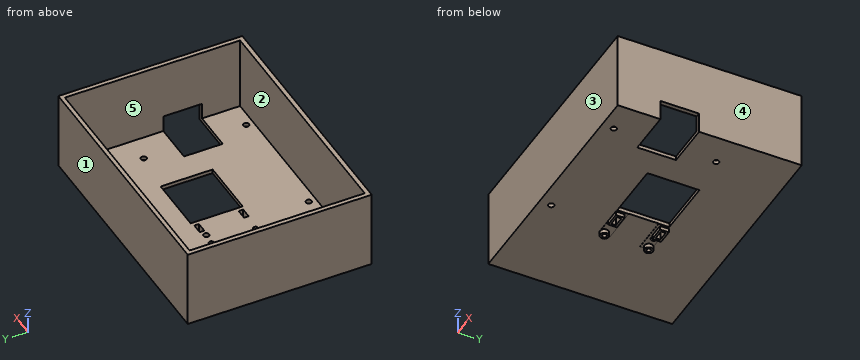
from build123d import *

# Parameters (mm, degrees)
SKETCH_1_W          = 120
SKETCH_1_H          = 80
EXTRUDE_1_DEPTH     = 38
SKETCH_3_W          = 117.6
SKETCH_3_H          = 77.6
CUT_EXTRUDE_1_DEPTH = 36
SKETCH_4_W          = 25.152970524
SKETCH_4_H          = 18.492901276
CUT_EXTRUDE_2_DEPTH = 10
SKETCH_7_W          = 17.413678367
SKETCH_7_H          = 5.076618726
SKETCH_7_H_2        = 5.541721388
EXTRUDE_2_DEPTH     = 0.1
SKETCH_9_W          = 27.882777132
SKETCH_9_H          = 24.878568111
CUT_EXTRUDE_4_DEPTH = 12
SKETCH_12_R         = 1.085209003
SKETCH_12_R_2       = 1.1
SKETCH_12_W         = 5.025
SKETCH_12_H         = 2.2
CUT_EXTRUDE_5_DEPTH = 12
SKETCH_13_R         = 1.35
CUT_EXTRUDE_6_DEPTH = 12
SKETCH_14_W         = 117.6
SKETCH_14_H         = 36
CUT_EXTRUDE_7_DEPTH = 10
EXTRUDE_3_DEPTH     = 5
SKETCH_16_W         = 120
SKETCH_16_H         = 38
EXTRUDE_4_DEPTH     = 2
SKETCH_17_W         = 36
SKETCH_17_H         = 83.8
EXTRUDE_5_DEPTH     = 1
EXTRUDE_6_DEPTH     = 1
SKETCH_19_W         = 120
SKETCH_19_H         = 38
EXTRUDE_7_DEPTH     = 1
EXTRUDE_START       = 2
SKETCH_20_R         = 2
SKETCH_20_R_2       = 1.085209003
SKETCH_20_R_3       = 2.001649737
SKETCH_20_R_4       = 1.1
SKETCH_20_W         = 7.2
SKETCH_20_H         = 4.2
SKETCH_20_W_2       = 5.025
SKETCH_20_H_2       = 2.2
EXTRUDE_8_DEPTH     = 2


with BuildPart() as part:
    # 草图1 → 凸台-拉伸1 (new body)
    with BuildSketch(Plane.XY):
        with Locations((-463.106796117, 303.186737633)):
            Rectangle(SKETCH_1_W, SKETCH_1_H)
    extrude(amount=EXTRUDE_1_DEPTH)

    # 草图3 → 切除-拉伸1 (cut)
    with BuildSketch(Plane.XY.offset(38)):
        with Locations((-463.106796117, 303.186737633)):
            Rectangle(SKETCH_3_W, SKETCH_3_H)
    extrude(amount=-CUT_EXTRUDE_1_DEPTH, mode=Mode.SUBTRACT)

    # 草图4 → 切除-拉伸2 (cut)
    with BuildSketch(Plane(origin=(0, 0, 0), x_dir=(-1, 0, 0), z_dir=(0, 0, -1))):
        with Locations((411.924701676, 291.841861287)):
            Rectangle(SKETCH_4_W, SKETCH_4_H)
    extrude(amount=-CUT_EXTRUDE_2_DEPTH, mode=Mode.SUBTRACT)

    # 草图7 → 凸台-拉伸2 (add)
    with BuildSketch(Plane(origin=(0, 0, 0), x_dir=(-1, 0, 0), z_dir=(0, 0, -1))):
        with Locations((474.461956934, 316.64842827)):
            Rectangle(SKETCH_7_W, SKETCH_7_H)
        with Locations((474.461956934, 296.957598327)):
            Rectangle(SKETCH_7_W, SKETCH_7_H_2)
    extrude(amount=EXTRUDE_2_DEPTH)

    # 草图9 → 切除-拉伸4 (cut)
    with BuildSketch(Plane(origin=(0, 0, 0), x_dir=(-1, 0, 0), z_dir=(0, 0, -1))):
        with Locations((451.813729184, 306.747453577)):
            Rectangle(SKETCH_9_W, SKETCH_9_H)
    extrude(amount=-CUT_EXTRUDE_4_DEPTH, mode=Mode.SUBTRACT)

    # 草图12 → 切除-拉伸5 (cut)
    with BuildSketch(Plane(origin=(0, 0, -0.1), x_dir=(-1, 0, 0), z_dir=(0, 0, -1))):
        with Locations((481.368796117, 317.386737633)):
            Circle(SKETCH_12_R)
        with Locations((481.368796117, 296.186737633)):
            Circle(SKETCH_12_R_2)
        with Locations((470.281296117, 317.386737633)):
            Rectangle(SKETCH_12_W, SKETCH_12_H)
        with Locations((470.281296117, 296.186737633)):
            Rectangle(SKETCH_12_W, SKETCH_12_H)
    extrude(amount=-CUT_EXTRUDE_5_DEPTH, mode=Mode.SUBTRACT)

    # 草图13 → 切除-拉伸6 (cut)
    with BuildSketch(Plane.XY.offset(2)):
        with Locations((-475.806796117, 316.886737633)):
            Circle(SKETCH_13_R)
        with Locations((-417.806796117, 316.886737633)):
            Circle(SKETCH_13_R)
        with Locations((-417.806796117, 267.886737633)):
            Circle(SKETCH_13_R)
        with Locations((-475.806796117, 267.886737633)):
            Circle(SKETCH_13_R)
    extrude(amount=-CUT_EXTRUDE_6_DEPTH, mode=Mode.SUBTRACT)

    # 草图14 → 切除-拉伸7 (cut)
    with BuildSketch(Plane.XZ.offset(-341.986737633)):
        with Locations((-463.106796117, 20)):
            Rectangle(SKETCH_14_W, SKETCH_14_H)
    extrude(amount=-CUT_EXTRUDE_7_DEPTH, mode=Mode.SUBTRACT)

    # 草图15 → 凸台-拉伸3 (add)
    with BuildSketch(Plane(origin=(0, 343.186737633, 0), x_dir=(1, 0, 0), z_dir=(0, 1, 0))):
        Polygon((-521.906796117, -2), (-404.306796117, -2), (-404.306796117, -38), (-403.106796117, -38), (-403.106796117, 0), (-523.106796117, 0), (-523.106796117, -38), (-521.906796117, -38), align=None)
    extrude(amount=EXTRUDE_3_DEPTH)

    # 草图16 → 凸台-拉伸4 (add)
    with BuildSketch(Plane(origin=(0, 348.186737633, 0), x_dir=(1, 0, 0), z_dir=(0, 1, 0))):
        with Locations((-463.106796117, -19)):
            Rectangle(SKETCH_16_W, SKETCH_16_H)
    extrude(amount=EXTRUDE_4_DEPTH)

    # 草图17 → 凸台-拉伸5 (add)
    with BuildSketch(Plane(origin=(-521.906796117, 0, 0), x_dir=(0, 0, -1), z_dir=(1, 0, 0))):
        with Locations((-20, 306.286737633)):
            Rectangle(SKETCH_17_W, SKETCH_17_H)
    extrude(amount=EXTRUDE_5_DEPTH)

    # 草图18 → 凸台-拉伸6 (add)
    with BuildSketch(Plane.ZY.offset(404.306796117)):
        Polygon((10, 301.088311925), (10, 282.595410649), (2, 282.595410649), (2, 264.386737633), (38, 264.386737633), (38, 348.186737633), (2, 348.186737633), (2, 301.088311925), align=None)
    extrude(amount=EXTRUDE_6_DEPTH)

    # 草图19 → 凸台-拉伸7 (add)
    with BuildSketch(Plane.XZ.offset(-263.186737633)):
        with Locations((-463.106796117, 19)):
            Rectangle(SKETCH_19_W, SKETCH_19_H)
    extrude(amount=EXTRUDE_7_DEPTH)

    # 草图20 → 凸台-拉伸8 (add)
    # profile 1 of 4: a face of its own
    with BuildSketch(Plane(origin=(0, 0, -0.1), x_dir=(-1, 0, 0), z_dir=(0, 0, -1)).offset(EXTRUDE_START)):
        with Locations(Location((481.368796117, 317.386737633, 0), (0, 0, 115.841932763))):
            Circle(SKETCH_20_R)
        with Locations((481.368796117, 317.386737633)):
            Circle(SKETCH_20_R_2, mode=Mode.SUBTRACT)
    # profile 2 of 4: a face of its own
    with BuildSketch(Plane(origin=(0, 0, -0.1), x_dir=(-1, 0, 0), z_dir=(0, 0, -1)).offset(EXTRUDE_START)):
        with Locations(Location((481.368796117, 296.186737633, 0), (0, 0, 267.673619076))):
            Circle(SKETCH_20_R_3)
        with Locations((481.368796117, 296.186737633)):
            Circle(SKETCH_20_R_4, mode=Mode.SUBTRACT)
    # profile 3 of 4: a face of its own
    with BuildSketch(Plane(origin=(0, 0, -0.1), x_dir=(-1, 0, 0), z_dir=(0, 0, -1)).offset(EXTRUDE_START)):
        with Locations((470.395177276, 317.386737633)):
            Rectangle(SKETCH_20_W, SKETCH_20_H)
        with Locations((470.281296117, 317.386737633)):
            Rectangle(SKETCH_20_W_2, SKETCH_20_H_2, mode=Mode.SUBTRACT)
    # profile 4 of 4: a face of its own
    with BuildSketch(Plane(origin=(0, 0, -0.1), x_dir=(-1, 0, 0), z_dir=(0, 0, -1)).offset(EXTRUDE_START)):
        with Locations((470.325427447, 296.233937818)):
            Rectangle(SKETCH_20_W, SKETCH_20_H)
        with Locations((470.281296117, 296.186737633)):
            Rectangle(SKETCH_20_W_2, SKETCH_20_H_2, mode=Mode.SUBTRACT)
    extrude(amount=-EXTRUDE_8_DEPTH)


solid = part.part
CAD build for the part. Positions are in the model's coordinates, mm. Face numbers are marked on the shaded views. A direction names the side the tool comes from. Give positions to 0.01 mm unless a question says otherwise; leave off trailing zeros. Order: outer loops, then holes, each group sorted by start corner. A loop starts at its lowest first (then second) coordinate and runs counter-clockwise, first axis right, second up. Notation, with made-up numbers: (30, 63.25) - (36, 63.25) arc R24 cw to (36, 86.25) - close; hole circle Ø7 at (63, 79). An arc over 180 degrees is marked (long way). Write each question's results on one line, items separated by ' | '.
1. Pin check, flat tips, straight feed: pin 1 (1 mm diameter, centred on x = -481, y = 271, fed in from +Z); pin 2 (10 mm diameter, centred on x = -470, y = 276.5, fed in from -Z); pin 3 (1 mm diameter, centred on x = -470, z = -1, fed in from +Y). Stop position of each tip, or through.
Calculated:
pin 1: stops at z = 2 | pin 2: stops at z = 0 | pin 3: stops at y = 319.49
2. Saw through at D-D on x = -492. List the corners of the cut face in (y, z).
Calculated:
outline: (262.19, 0) - (350.19, 0) - (350.19, 38) - (348.19, 38) - (348.19, 2) - (264.39, 2) - (264.39, 38) - (262.19, 38) - close
3. 3-axis set-ups, long thin cutter, end or side, ignore diameter. For the marked faces 1 and 2: which of +Z, -Z, +X, -X, +Y, -Y reach the whole face in a straight line?
Calculated:
face 1: +Z, -Z, +X, -X, +Y | face 2: +Z
4. Saw through at C-C on z = 31. List the corners of the cut face in (x, y).
Calculated:
outline: (-523.11, 262.19) - (-403.11, 262.19) - (-403.11, 350.19) - (-523.11, 350.19) - close; hole (-520.91, 264.39) - (-405.31, 264.39) - (-405.31, 348.19) - (-520.91, 348.19) - close
5. Pull direction X, two halves, no side cores. Call the marked faces 3, 4 and 5: released by +X, released by -X, zero draft, split by the parting line, or undercut.
Calculated:
face 3: zero draft | face 4: released by +X | face 5: undercut
6. Saw through at A-A on y = 303.5. List the corners of the cut face in (x, z).
Calculated:
outline: (-523.11, 0) - (-465.76, 0) - (-465.76, 2) - (-520.91, 2) - (-520.91, 38) - (-523.11, 38) - close; (-437.87, 0) - (-403.11, 0) - (-403.11, 38) - (-405.31, 38) - (-405.31, 2) - (-437.87, 2) - close
7. Probe L1, parallel to X at y = 286, z = 13.5; L2, parallel to Y at x = -467.5, z = 28; L3, parallel to Z at x = -484.5, y = 270. List the from-to ranges inside material, lowest first. Write a range as from..to.
Calculated:
L1: x = -523.11..-520.91, -405.31..-403.11 | L2: y = 262.19..264.39, 348.19..350.19 | L3: z = 0..2
8. Saw through at B-B on x = -415. List the corners of the cut face in (y, z), and give its area (3 significant figures).
Calculated:
outline: (262.19, 0) - (282.6, 0) - (282.6, 2) - (264.39, 2) - (264.39, 38) - (262.19, 38) - close; (301.09, 0) - (350.19, 0) - (350.19, 38) - (348.19, 38) - (348.19, 2) - (301.09, 2) - close | area: 290 mm2
